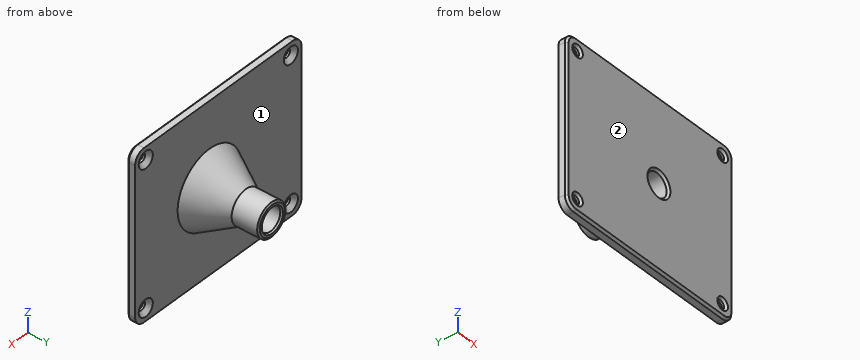
```python
from build123d import *
from OCP.BRepFilletAPI import BRepFilletAPI_MakeChamfer

# Parameters (mm, degrees)
SKETCH_1_W          = 94
SKETCH_1_H          = 80
SKETCH_1_R          = 2
EXTRUDE_1_DEPTH     = 4
FILLET_1_R          = 5
SKETCH_2_R          = 8
EXTRUDE_2_DEPTH     = 30
SKETCH_3_R          = 5.5
CUT_EXTRUDE_1_DEPTH = 71.46275612
CHAMFER_1_SIZE      = 1
CHAMFER_2_SIZE      = 10
CHAMFER_2_SIZE2     = 17.320508076
CHAMFER_3_SIZE      = 2
CHAMFER_4_SIZE      = 0.5
CHAMFER_4_SIZE2     = 0.866025404


with BuildPart() as part:
    # Эскиз1 → Бобышка-Вытянуть1 (new body)
    with BuildSketch(Plane(origin=(0, 0, 0), x_dir=(1, 0, 0), z_dir=(0, 1, 0))):
        Rectangle(SKETCH_1_W, SKETCH_1_H)
        with Locations(Location((41, 34, 0), (0, 0, 270))):
            Circle(SKETCH_1_R, mode=Mode.SUBTRACT)
        with Locations(Location((-41, 34, 0), (0, 0, 90))):
            Circle(SKETCH_1_R, mode=Mode.SUBTRACT)
        with Locations(Location((-41, -34, 0), (0, 0, 270))):
            Circle(SKETCH_1_R, mode=Mode.SUBTRACT)
        with Locations(Location((41, -34, 0), (0, 0, 90))):
            Circle(SKETCH_1_R, mode=Mode.SUBTRACT)
    extrude(amount=EXTRUDE_1_DEPTH)

    # Скругление1
    fillet_1_edges = [part.edges().sort_by_distance(p)[0] for p in [
        (47, 2, 40),
        (-47, 2, 40),
        (-47, 2, -40),
        (47, 2, -40),
    ]]
    fillet(fillet_1_edges, radius=FILLET_1_R)

    # Эскиз2 → Бобышка-Вытянуть2 (add)
    with BuildSketch(Plane(origin=(0, 4, 0), x_dir=(1, 0, 0), z_dir=(0, 1, 0))):
        with Locations(Location((5, 0, 0), (0, 0, 270))):
            Circle(SKETCH_2_R)
    extrude(amount=EXTRUDE_2_DEPTH)

    # Эскиз3 → Вырез-Вытянуть1 (cut, through all)
    with BuildSketch(Plane(origin=(0, 34, 0), x_dir=(1, 0, 0), z_dir=(0, 1, 0))):
        with Locations(Location((5, 0, 0), (0, 0, 270))):
            Circle(SKETCH_3_R)
    extrude(amount=-CUT_EXTRUDE_1_DEPTH, mode=Mode.SUBTRACT)

    # Фаска1
    chamfer_1_edges = [part.edges().sort_by_distance(p)[0] for p in [
        (41, 0, -36),
        (-41, 0, -32),
        (-41, 0, 32),
        (41, 0, 36),
        (0, 0, 40),
        (47, 0, 0),
        (-47, 0, 0),
        (0, 0, -40),
        (45.535533906, 0, 38.535533906),
        (45.535533906, 0, -38.535533906),
        (-45.535533906, 0, -38.535533906),
        (-45.535533906, 0, 38.535533906),
        (5, 0, -5.5),
    ]]
    chamfer(chamfer_1_edges, length=CHAMFER_1_SIZE)

    # Фаска2
    chamfer_2_edges = [part.edges().sort_by_distance(p)[0] for p in [
        (5, 4, -8),
    ]]
    chamfer_2_side = [part.faces().sort_by_distance(p)[0] for p in [
        (0, 4, 38.76565807),
    ]]
    chamfer(chamfer_2_edges, length=CHAMFER_2_SIZE, length2=CHAMFER_2_SIZE2, reference=chamfer_2_side[0])

    # Фаска3
    chamfer_3_edges = [part.edges().sort_by_distance(p)[0] for p in [
        (41, 4, -36),
        (-41, 4, -32),
        (-41, 4, 32),
        (41, 4, 36),
    ]]
    chamfer(chamfer_3_edges, length=CHAMFER_3_SIZE)

    # Фаска4: one chamfer whose edges measure the first distance from different faces: ONE call of the kernel's chamfer builder (chamfer() names one face for all edges)
    chamfer_4_edges_1 = [part.edges().sort_by_distance(p)[0] for p in [
        (5, 34, -8),
    ]]
    chamfer_4_side_1 = [part.faces().sort_by_distance(p)[0] for p in [
        (5, 27.660254038, -8),
    ]]
    chamfer_4_edges_2 = [part.edges().sort_by_distance(p)[0] for p in [
        (5, 34, -5.5),
    ]]
    chamfer_4_side_2 = [part.faces().sort_by_distance(p)[0] for p in [
        (5, 34, -7.77372583),
    ]]
    chamfer_4 = BRepFilletAPI_MakeChamfer(part.part.solid().wrapped)
    for e in chamfer_4_edges_1:
        chamfer_4.Add(CHAMFER_4_SIZE, CHAMFER_4_SIZE2, e.wrapped, chamfer_4_side_1[0].wrapped)  # the first distance lies on this face
    for e in chamfer_4_edges_2:
        chamfer_4.Add(CHAMFER_4_SIZE, CHAMFER_4_SIZE2, e.wrapped, chamfer_4_side_2[0].wrapped)  # the first distance lies on this face
    add(Compound.cast(chamfer_4.Shape()), mode=Mode.REPLACE)


solid = part.part
```
Verification items for the finished model (mm, model axes). Face numbers are marked on the shaded views. A direction names the side the tool comes from. Coordinates: 2 decimals unless noted, no trailing zeros. Loops run counter-clockwise (first coordinate to the right, second up) from the corner with the lowest first, then second, coordinate; pieces in that order, holes last. Notation, with made-up numbers: (53.5, 68.5) -> (60.5, 68.5) arc R25 ccw to (60.5, 100.5) -> close; hole circle Ø7 at (-35, -15.75). An arc over 180 degrees is marked (long way). Answer in a Markdown table with one row per item. Add a question column.
1. Depth check by flat-ended pin: P1, Ø4, axis at x = -6.5, y = 23, coming from the -Z side; P2, Ø5, axis at x = 41, z = -34, coming from the -Y side; P3, Ø4, axis at x = -27.5, z = 9, coming from the +Y side; P4, Ø1, axis at x = -3.5, z = -8, coming from the -Y side. Enter the tip coordinate at first touch or a pass-through.
2. Material ranges on probe 1 along X at (y, z) = (1, 34); probe 2 along X at (y, z) = (21.5, 0); probe 3 along Y at (x, z) = (-42, -27.5), recorded low to high. Write a range as [from, to].
3. Section check B-B, the plane x = 24.5. Enter the section's corners in (y, z), then the cut area to 3 significant figures.
4. Section check D-D, the plane y = 6.5. Enter the section's corners in (x, z).
5. Section check A-A, the plane z = 23.5. Enter the section's corners in (x, y).
6. Section check C-C, the plane y = 29. Enter the section's corners in (x, z), then the cut area to 3 significant figures.
7. Access from +Z, -Z, +X, -X, +Y, -Y to the whole of each face (thin tool, end or side, straight path). Record for the marked faces 1 and 2.
Derived:
| question | item | result |
|---|---|---|
| 1 | P1 | passes through |
| 1 | P2 | stops at y = 0.5 |
| 1 | P3 | stops at y = 4 |
| 1 | P4 | stops at y = 0 |
| 2 | probe 1 | x = [-47, -43], [-39, 39], [43, 47] |
| 2 | probe 2 | x = [-3, -0.5], [10.5, 13] |
| 2 | probe 3 | y = [0, 4] |
| 3 | outline | (0, -39) -> (1, -40) -> (4, -40) -> (4, 40) -> (1, 40) -> (0, 39) -> close |
| 3 | area | 319 mm² |
| 4 | outline | circle Ø33.11 at (5, 0); hole circle Ø11 at (5, 0) |
| 5 | outline | (-47, 1) -> (-46, 0) -> (46, 0) -> (47, 1) -> (47, 4) -> (-47, 4) -> close |
| 6 | outline | circle Ø16 at (5, 0); hole circle Ø11 at (5, 0) |
| 6 | area | 106 mm² |
| 7 | face 1 | +Y |
| 7 | face 2 | +Z, -Z, +X, -X, -Y |
